For this review, use the dimensioned drawing (mm, ordinates from the lowest corner) and the shaded views. Give positions to 0.01 mm unless a question says otherwise; leave off trailing zeros. Loops run counter-clockwise (first coordinate to the right, second up) from the corner with the lowest first, then second, coordinate; pieces in that order, holes last. Notation, with made-up numbers: (74.25, 62) -> (106.25, 62) arc R9 ccw to (106.25, 73) -> close; hole circle Ø4 at (60.5, -7.75). An arc over 180 degrees is marked (long way). Use a Markdown table: item, result. Add a question column.
1. Add section B-B (x = 16). State the section outline as (y, z) points.
2. To check wall thickness, follow line 1 (Z direction, x = 9, y = 0.3); line 2 (Z direction, x = 121.5, y = 1); line 3 (X direction, y = 1.05, z = 27). State the ranges of each line that lie inside material, in increasing order.
3. Add section A-A (y = 0.9). State the section outline as (x, z) points, and give its area (3 significant figures).
4. Add section C-C (z = 14.5). State the section outline as (x, y) points.
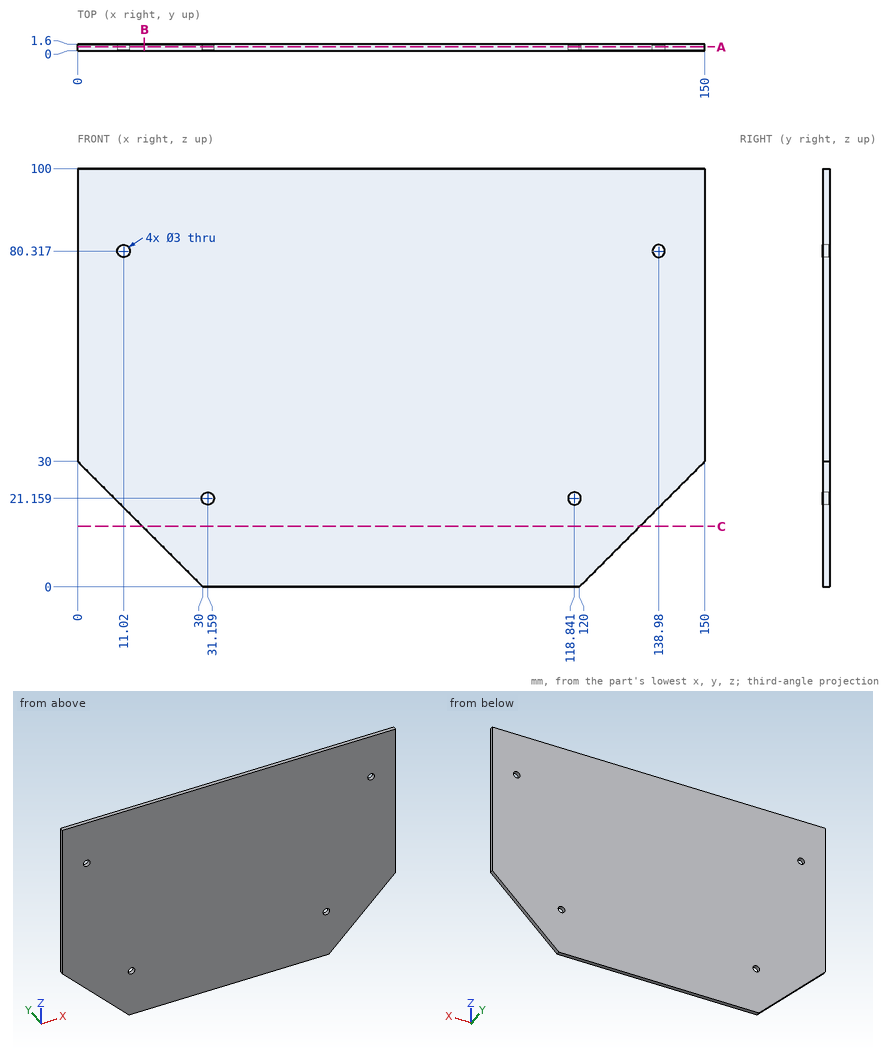
Taken from the geometry:
| question | item | result |
|---|---|---|
| 1 | outline | (0, 14) -> (1.6, 14) -> (1.6, 100) -> (0, 100) -> close |
| 2 | line 1 | z = 21 to 100 |
| 2 | line 2 | z = 1.5 to 100 |
| 2 | line 3 | x = 3 to 147 |
| 3 | outline | (0, 30) -> (30, 0) -> (120, 0) -> (150, 30) -> (150, 100) -> (0, 100) -> close; hole circle Ø3 at (11.02, 80.32); hole circle Ø3 at (31.16, 21.16); hole circle Ø3 at (118.84, 21.16); hole circle Ø3 at (138.98, 80.32) |
| 3 | area | 14,100 mm^2 |
| 4 | outline | (15.5, 0) -> (134.5, 0) -> (134.5, 1.6) -> (15.5, 1.6) -> close |
